```python
from build123d import *

# Parameters (mm, degrees)
F0_W      = 65
F0_H      = 65
F1_DEPTH  = 8
F2_W      = 65
F2_H      = 20
F3_DEPTH  = 8
F4_W      = 60
F4_H      = 3.6
F5_DEPTH  = 15
F6_R      = 3.99999
F7_W      = 65
F7_H      = 8
F8_DEPTH  = 14
F9_W      = 65
F9_H      = 8
F10_DEPTH = 12
F11_R     = 3.99999


# Not quite as in the source:
# - a fillet or chamfer is up to 0.001 mm smaller than in the source, because OpenCascade refuses the exact size


with BuildPart() as f1:
    # F0 (on Top) → F1 (new body)
    with BuildSketch(Plane.XY):
        Rectangle(F0_W, F0_H)
    extrude(amount=F1_DEPTH)

    # F2 (on face) → F3 (join)
    with BuildSketch(Plane.XZ.offset(32.5)):
        with Locations((0, -2)):
            Rectangle(F2_W, F2_H)
    extrude(amount=-F3_DEPTH)

    # F4 (on face) → F5 (join)
    with BuildSketch(Plane(origin=(0, 32.5, 0), x_dir=(-1, 0, 0), z_dir=(0, 1, 0))):
        with Locations((0, 4)):
            Rectangle(F4_W, F4_H)
    extrude(amount=F5_DEPTH)

    # F6 (radius 4 in the source; OpenCascade refuses exactly that, so slightly less here)
    f6_edges = [f1.edges().sort_by_distance(p)[0] for p in [
        (-32.5, -24.5, -6),
        (-32.5, -32.5, -2),
        (32.5, -24.5, -6),
        (32.5, -32.5, -2),
        (32.5, 0, 8),
        (-32.5, 0, 8),
        (32.5, 4, 0),
        (-32.5, 4, 0),
    ]]
    fillet(f6_edges, radius=F6_R)

    # F7 (on face) → F8 (join)
    with BuildSketch(Plane(origin=(0, 47.5, 0), x_dir=(-1, 0, 0), z_dir=(0, 1, 0))):
        with Locations((0, 4)):
            Rectangle(F7_W, F7_H)
    extrude(amount=F8_DEPTH)

    # F9 (on face) → F10 (join, through all)
    with BuildSketch(Plane(origin=(0, 0, 0), x_dir=(1, 0, 0), z_dir=(0, 0, -1))):
        with Locations((0, -57.5)):
            Rectangle(F9_W, F9_H)
    extrude(amount=F10_DEPTH)

    # F11 (radius 4 in the source; OpenCascade refuses exactly that, so slightly less here)
    f11_edges = [f1.edges().sort_by_distance(p)[0] for p in [
        (-32.5, 61.5, -2),
        (-32.5, 53.5, -6),
        (-32.5, 50.5, 0),
        (-32.5, 54.5, 8),
        (32.5, 50.5, 0),
        (32.5, 54.5, 8),
        (32.5, 61.5, -2),
        (32.5, 53.5, -6),
    ]]
    fillet(f11_edges, radius=F11_R)


solid = f1.part
```
The listing builds one solid part. Answer for the finished solid, in the listing's coordinates (mm). A direction names the side the tool comes from. Give positions to 0.01 mm unless a question says otherwise; leave off trailing zeros. Order: outer loops, then holes, each group sorted by start corner. A loop starts at its lowest first (then second) coordinate and runs counter-clockwise, first axis right, second up. Notation, with made-up numbers: (54.25, -13.75) - (60.25, -13.75) arc R20 cw to (60.25, 3.25) - close; hole circle Ø9 at (9.5, 2). An arc over 180 degrees is marked (long way). Use one line per item in the form item = value. Start each with the question number.
(1) The mould has two halves that part along Y. Classify faces 1 (the flat face through (0, 0, 8)), 2 (the flat face through (0, 61.5, -2)), 3 (the cylindrical face through (-31.359, 2.427, 1.203)): released by +Y, released by -Y, zero draft, split by the parting line, or undercut.
(2) Consider line 1 (Y direction, x = -10, z = -3.5); line 2 (Y direction, x = 6.5, z = 0.75); line 3 (Z direction, x = 26.5, y = -7.5). Determine where each line is inside the solid, lowest interval first. Write a range as from..to.
(3) Flat-ended cylindrical pins translate along their axes: pin 1 Ø8 at (y, z) = (-11, -1.5) entering from +X; pin 2 Ø7.5 at (x, y) = (-8.5, 43) entering from +Z; pin 3 Ø4 at (y, z) = (36.5, 3.5) entering from +X. Find the tip coordinate at first contact, or state that the pin passes through.
(4) For faces 4 (the cylindrical face through (-31.359, 0.455, 6.797)), 5 (the cylindrical face through (-31.359, -25.703, -5.666)), 6 (the flat face through (0, 4, 0)), 7 (the cylindrical face through (31.359, 51.459, 1.203)), 8 (the flat face through (0, 57, -12)), determine the directions among +Z, -Z, +X, -X, +Y, -Y from which every point of the face is accessible in a straight line to the end or side of a thin tool.
(5) A cutting plane is placed at D-D, the plane y = 46. Write down the section's boundary in (x, z), then the cut area to 3 significant figures.
(6) A cutting plane is placed at C-C, the plane x = 11.5. Write down the section's boundary in (y, z), then the cut area to 3 significant figures.
Ans:
q1.face_1 = zero draft
q1.face_2 = released by +Y
q1.face_3 = undercut
q2.line_1 = -32.5..-24.5, 53.5..61.5
q2.line_2 = -32.5..32.5, 47.5..61.5
q2.line_3 = 0..8
q3.pin_1 = 32.21
q3.pin_2 = 5.8
q3.pin_3 = 30
q4.face_4 = +Z, -X, +Y, -Y
q4.face_5 = -Z, -X
q4.face_6 = -Z, +X, -X
q4.face_7 = -Z, +X
q4.face_8 = -Z, +X, -X, +Y, -Y
q5.outline = (-30, 2.2) - (30, 2.2) - (30, 5.8) - (-30, 5.8) - close
q5.area = 216 mm^2
q6.outline = (-32.5, -12) - (-24.5, -12) - (-24.5, 0) - (32.5, 0) - (32.5, 2.2) - (47.5, 2.2) - (47.5, 0) - (53.5, 0) - (53.5, -12) - (61.5, -12) - (61.5, 8) - (47.5, 8) - (47.5, 5.8) - (32.5, 5.8) - (32.5, 8) - (-32.5, 8) - close
q6.area = 878 mm^2
